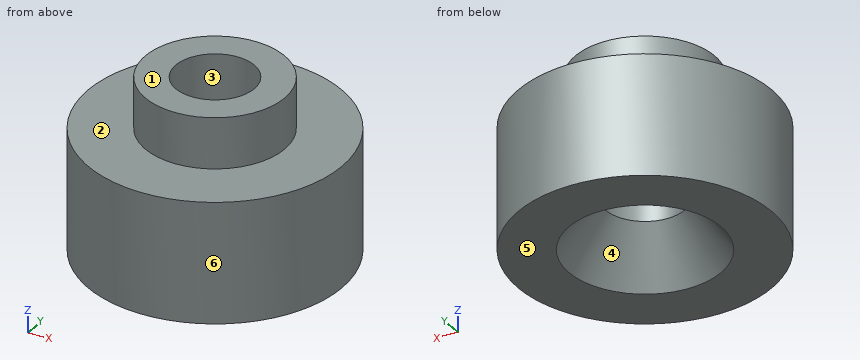
```python
from build123d import *

# Parameters (mm, degrees)
SKETCH_1_R      = 5
SKETCH_1_R_2    = 1.55
EXTRUDE_1_DEPTH = 4.75
SKETCH_2_R      = 2.75
SKETCH_2_R_2    = 1.55
EXTRUDE_2_DEPTH = 2


with BuildPart() as part:
    # 草图1 → 凸台-拉伸1 (new body)
    with BuildSketch(Plane.XY):
        Circle(SKETCH_1_R)
        Circle(SKETCH_1_R_2, mode=Mode.SUBTRACT)
    extrude(amount=EXTRUDE_1_DEPTH)

    # 草图2 → 凸台-拉伸2 (add)
    with BuildSketch(Plane.XY.offset(4.75)):
        Circle(SKETCH_2_R)
        Circle(SKETCH_2_R_2, mode=Mode.SUBTRACT)
    extrude(amount=EXTRUDE_2_DEPTH)

    # 草图5 → 切除-旋转1 (revolve, cut)
    with BuildSketch(Plane(origin=(0, 0, 0), x_dir=(1, 0, 0), z_dir=(0, 1, 0))):
        Polygon((3, 0), (1.55, -2), (0, -2), (0, 0), align=None)
    revolve(axis=Axis((0, 0, 4.75), (0, 0, -1)), mode=Mode.SUBTRACT)


solid = part.part
```
Input: part model. Units: mm. Frame: model coordinates. Face numbers are marked on the shaded views. A direction names the side the tool comes from. Round coordinates to 2 decimals unless told otherwise and drop trailing zeros. Loops run counter-clockwise (first coordinate to the right, second up) from the corner with the lowest first, then second, coordinate; pieces in that order, holes last. Notation, with made-up numbers: (60, 33.5) -> (80, 33.5) arc R14 cw to (80, 44.5) -> close; hole circle Ø1 at (-6.75, 68.5). An arc over 180 degrees is marked (long way). One line per item, written item: value.
(1) Section D-D (x = 4). Return the cut outline in (y, z), plus the area to 3 significant figures.
Geometry check:
outline: (-3, 0) -> (3, 0) -> (3, 4.75) -> (-3, 4.75) -> close
area: 28.5 mm2
(2) Section A-A (y = 0). Return the cut outline in (x, z), plus the area to 3 significant figures.
Geometry check:
outline: (-5, 0) -> (-3, 0) -> (-1.55, 2) -> (-1.55, 6.75) -> (-2.75, 6.75) -> (-2.75, 4.75) -> (-5, 4.75) -> close; (1.55, 2) -> (3, 0) -> (5, 0) -> (5, 4.75) -> (2.75, 4.75) -> (2.75, 6.75) -> (1.55, 6.75) -> close
area: 34.7 mm2
(3) Section C-C (z = 6). Return the cut outline in (x, y).
Geometry check:
outline: circle Ø5.5 at (0, 0); hole circle Ø3.1 at (0, 0)
(4) Material intervals for line 1 (Y direction, x = 0, z = 4.6); line 2 (Y direction, x = 0, z = 5.85); line 3 (Z direction, x = 0.5, y = -3), sorted ascending. Write a range as [from, to].
Geometry check:
line 1: [-5, -1.55], [1.55, 5]
line 2: [-2.75, -1.55], [1.55, 2.75]
line 3: [0, 4.75]
(5) Mould query, pull axis X, two halves, no side actions, for the marked faces 3, 4, 5 and 6. Classes: pulls with the +X half, pulls with the -X half, needs draft (parallel to the pull), parting line crosses it, or undercut.
Geometry check:
face 3: undercut
face 4: undercut
face 5: needs draft
face 6: parting line crosses it
(6) Set-up query: the marked faces 1 and 2. Return all of +Z, -Z, +X, -X, +Y, -Y with unobstructed straight access to the full face (end or side cutting, diameter ignored); none if empty.
Geometry check:
face 1: +Z, +X, -X, +Y, -Y
face 2: +Z
(7) Pin query (flat end, axial travel): pin 1 (5 mm diameter, centred on x = 0, y = 0, fed in from +Z); pin 2 (3 mm diameter, centred on x = -2.5, z = 2, fed in from +Y); pin 3 (3 mm diameter, centred on x = 2, z = 5, fed in from +Y). Return the tip coordinate at first contact, or that it passes through.
Geometry check:
pin 1: z = 6.75
pin 2: y = 4.9
pin 3: y = 4.97
